Autodesk Inventor part; units mm, degrees
ref_plane "Work Plane1" through (0, 20, 0) normal (0, -1, 0) x (1, 0, 0)
ref_plane "YZ Plane" through (0, 0, 0) normal (1, 0, 0) x (0, 1, 0)
ref_plane "XZ Plane" through (0, 0, 0) normal (0, 1, 0) x (-1, 0, 0)
sketch "Sketch1" plane through (0, 0, 0) normal (0, 1, 0) x (-1, 0, 0)
  line L0 (-19.05, -19.05) -> (19.05, -19.05) construction
  line L1 (19.05, -19.05) -> (19.05, 19.05) construction
  line L2 (19.05, 19.05) -> (-19.05, 19.05) construction
  line L3 (-19.05, 19.05) -> (-19.05, -19.05) construction
  line L4 (-19.05, -19.05) -> (19.05, 19.05) construction
  line L5 (19.05, -19.05) -> (-19.05, 19.05) construction
  line L6 (-19.05, 19.05) -> (19.05, 19.05) construction
  line L7 (19.05, 19.05) -> (19.05, 39.05) construction
  line L8 (19.05, 39.05) -> (-19.05, 39.05)
  line L9 (-19.05, 39.05) -> (-19.05, 19.05) construction
  line L10 (19.05, 39.05) -> (39.05, 39.05)
  line L11 (39.05, 39.05) -> (39.05, -19.05)
  line L12 (39.05, -19.05) -> (19.05, -19.05) construction
  line L13 (19.05, -19.05) -> (19.05, 19.05) construction
  line L14 (19.05, 19.05) -> (19.05, 39.05) construction
  line L15 (-19.05, 39.05) -> (39.05, 39.05)
  line L16 (45.4, 39.05) -> (45.4, 45.4)
  line L17 (45.4, 45.4) -> (-19.05, 45.4)
  line L18 (-19.05, 45.4) -> (-19.05, 39.05)
  line L19 (45.4, 39.05) -> (39.05, 39.05) construction
  line L20 (39.05, 39.05) -> (39.05, -19.05)
  line L21 (39.05, -19.05) -> (45.4, -19.05)
  line L22 (45.4, -19.05) -> (45.4, 39.05)
  line L23 (39.05, 39.05) -> (45.4, 39.05) construction
  point P0 (0, 0)
  dimension "d0" = 38.1
  dimension "d1" = 20
  dimension "d2" = 20
  dimension "d3" = 6.35
  dimension "d4" = 6.35
  dimension "d67" = 0
extrude "Extrusion1" add sketch "Sketch1" along normal blind 62.3
sketch "Sketch2" plane through (-45.4, 0, 45.4) normal (0, 0, 1) x (1, 0, 0)
  line L0 (6.35, 0) -> (0, 0)
  line L1 (64.45, 0) -> (64.45, 62.3)
  line L2 (0, 0) -> (64.45, 0)
  line L3 (64.45, 0) -> (64.45, 20)
  line L4 (64.45, 20) -> (0, 20)
  line L5 (0, 20) -> (0, 0)
  line L6 (0, 0) -> (0, 62.3)
  line L7 (0, 10) -> (64.45, 10) construction
  circle A0 centre (19.05, 10) radius 2.75
  circle A1 centre (35.4, 10) radius 2.75
  circle A2 centre (51.75, 10) radius 2.75
  point P0 (45.4, 0)
  dimension "d7" = 20
  dimension "d8" = 5.5
  dimension "d12" = 16.35
  dimension "d68" = 12.7
extrude "Extrusion2" cut sketch "Sketch2" against normal blind 62.3 contours A0 | A1 | A2
sketch "Sketch3" plane through (-45.4, 0, -19.05) normal (-1, 0, 0) x (0, 0, 1)
  circle A0 centre (12.7, 10) radius 2.75
  line L0 (0, 0) -> (64.45, 0)
  line L1 (0, 0) -> (0, 62.3)
  circle A1 centre (29.05, 10) radius 2.75
  circle A2 centre (45.4, 10) radius 2.75
  point P0 (19.05, 0)
  dimension "d19" = 10
  dimension "d20" = 5.5
  dimension "d21" = 12.7
  dimension "d24" = 16.35
extrude "Extrusion3" cut sketch "Sketch3" against normal blind 62.3
ref_plane "Work Plane1" through (0, 20, 0) normal (0, -1, 0) x (1, 0, 0)
sketch "Sketch4" plane through (0, 20, 0) normal (0, -1, 0) x (1, 0, 0)
  line L0 (-39.05, -19.05) -> (-45.4, -19.05)
  line L1 (-39.05, 39.05) -> (-39.05, -19.05)
  line L2 (19.05, 39.05) -> (-39.05, 39.05)
  line L3 (19.05, 45.4) -> (19.05, 39.05)
  line L4 (-45.4, 45.4) -> (19.05, 45.4)
  line L5 (-45.4, -19.05) -> (-45.4, 45.4)
  line L6 (-39.05, 39.05) -> (-39.05, -19.05)
  line L7 (-39.05, 39.05) -> (-19.05, 39.05)
  line L8 (-19.05, 39.05) -> (-19.05, 19.05) construction
  line L9 (-19.05, -19.05) -> (-39.05, -19.05)
  line L10 (-39.05, -19.05) -> (-39.05, 39.05)
  line L11 (19.05, 39.05) -> (-39.05, 39.05)
  line L12 (19.05, 39.05) -> (-19.05, 39.05)
  line L13 (-19.05, 39.05) -> (-19.05, 19.05) construction
  line L14 (-19.05, 19.05) -> (19.05, 19.05) construction
  line L15 (19.05, 19.05) -> (19.05, 39.05)
  line L16 (-19.05, 19.05) -> (-19.05, -19.05) construction
  line L17 (19.05, 29.05) -> (-39.05, 29.05) construction
  line L18 (-29.05, -19.05) -> (-29.05, 39.05) construction
  circle A0 centre (-29.05, 29.05) radius 2.75
  circle A1 centre (-10, 29.05) radius 2.75
  circle A2 centre (9.05, 29.05) radius 2.75
  circle A3 centre (-29.05, 10) radius 2.75
  circle A4 centre (-29.05, -9.05) radius 2.75
  line L19 (19.05, 19.05) -> (19.05, 12.7)
  line L20 (19.05, 12.7) -> (-19.05, -19.05)
  circle A5 centre (-29.05, 4.126) radius 2.7544
  point P0 (0, 0)
  dimension "d32" = 20
  dimension "d35" = 19.05
  dimension "d40" = 5.5
  dimension "d43" = 19.05
  dimension "d50" = 6.35
  dimension "d69" = 0
extrude "Extrusion4" add sketch "Sketch4" against normal blind 6.35 contours L1 L2 L15 L19 L20 L9 | A3
sketch "Sketch5" plane through (0, 26.35, 0) normal (0, 1, 0) x (1, 0, 0)
  line L0 (19.05, -39.05) -> (19.05, -12.7)
  line L1 (-39.05, -39.05) -> (-39.05, 19.05)
  line L2 (19.05, -12.7) -> (-39.05, -12.7)
  line L3 (-39.05, -12.7) -> (-39.05, -19.05)
  line L4 (-39.05, -19.05) -> (19.05, -19.05)
  line L5 (19.05, -19.05) -> (19.05, -12.7)
  point P0 (0, 0)
  dimension "d51" = 6.35
extrude "Extrusion5" add sketch "Sketch5" along normal up to surface (35.95 mm away)
sketch "Sketch7" plane through (-39.05, 26.35, -19.05) normal (1, 0, 0) x (0, 0, -1)
  line L0 (-31.75, 35.95) -> (0, 35.95)
  line L1 (-31.75, 35.95) -> (0, 35.95)
  line L2 (0, 0) -> (0, 35.95)
  line L3 (0, 35.95) -> (0, 0)
  line L4 (0, 0) -> (-31.75, 35.95)
  point P0 (-19.05, -26.35)
extrude "Extrusion7" cut sketch "Sketch7" against normal through all
sketch "Sketch8" plane through (-45.4, 0, 45.4) normal (0, 0, 1) x (1, 0, 0)
  line L0 (64.45, 62.3) -> (6.35, 62.3)
  line L1 (6.35, 26.35) -> (6.35, 62.3)
  line L2 (64.45, 26.35) -> (6.35, 26.35)
  line L3 (64.45, 26.35) -> (64.45, 62.3)
  line L4 (64.45, 20) -> (64.45, 26.35)
  line L5 (6.35, 62.3) -> (64.45, 26.35)
  line L6 (6.35, 62.3) -> (64.45, 62.3)
  line L7 (64.45, 26.35) -> (64.45, 62.3)
  line L8 (64.45, 62.3) -> (6.35, 62.3)
  point P0 (45.4, 0)
extrude "Extrusion8" cut sketch "Sketch8" against normal through all contours L3 L5 L0
sketch "Sketch9" plane through (-39.05, 26.35, 39.05) normal (1, 0, 0) x (0, 0, -1)
  line L0 (12.75, -6.35) -> (7.25, -6.35)
  line L1 (10, -6.35) -> (10, 18.61)
  circle A0 centre (10, 18.61) radius 2.75
  point P0 (39.05, -26.35)
  dimension "d63" = 24.96
  dimension "d64" = 5.5
extrude "Extrusion9" cut sketch "Sketch9" against normal through all
properties part number "xIdler"
The model under review builds one solid part; all positions refer to its coordinate system, in mm. A direction names the side the tool comes from. Give positions to 0.01 mm unless a question says otherwise; leave off trailing zeros. Write each loop counter-clockwise with the first axis right and the second up, starting at its lowest first coordinate (ties: lowest second). Pieces come first, ordered by that corner, then holes. Notation, with made-up numbers: M 48,24 L 89,24 A26 cw 89,43 Z; hole C -18.5,89 d8. An arc over 180 degrees is marked long. Write each question's results on one line, items separated by ' | '. Start each with the question number.
1. We need section D-D (x = -22.5). Write out the cut boundary in (y, z).
2. We need section B-B (y = 24). Write out the cut boundary in (x, z), and give its area (3 significant figures).
3. We need section C-C (y = 15.5). Write out the cut boundary in (x, z), and give its area (3 significant figures).
4. We need section A-A (z = -10). Write out the cut boundary in (x, y), and give its area (3 significant figures).
5. Mouldability with a two-part tool opening along Z and no side actions: class faces 5 (the flat face through (-25, 0, 40)), 6 (the flat face through (-23, 36, 12.7)), 7 (the cylindrical face through (-8.52, 23.13, 31.37)) as released by +Z, released by -Z, zero draft, split by the parting line, or undercut.
6. For probe 1 along Z at (x, y) = (-29.05, 23.75); probe 2 along X at (y, z) = (22, 29); probe 3 along Z at (x, y) = (-19.5, 31), list the stretches that pass through material, from the lowest coordinate up. Write a range as [from, to].
7. Insertion check: pin 1 Ø3.5 at (x, z) = (-10, 29.05) entering from +Y; pin 2 Ø10 at (x, z) = (-18, 4) entering from -Y; pin 3 Ø16 at (y, z) = (13, -1) entering from +X; pin 4 Ø6.5 at (x, z) = (-29.05, 29.05) entering from +Y. Each pin has a flat end and moves straight along its axis. Give the tip position at first contact, or say it passes through.
8. For faces 1 (the flat face through (-39.05, 40, 29)), 2 (the flat face through (-39.05, 40, 1)), 3 (the flat face through (-10, 5, 39.05)), 4 (the flat face through (-10.41, 44.58, 15.92)), list the 3-axis set-ups (+Z, -Z, +X, -X, +Y, -Y) from which the entire face can be reached by the end or side of a thin tool; tool diameter is ignored.
Results found:
1) outline: M 0,39.05 L 20,39.05 L 20,-19.05 L 26.35,-19.05 L 26.35,12.7 L 52.06,12.7 L 52.06,19.05 L 26.35,19.05 L 26.35,39.05 L 52.06,39.05 L 52.06,45.4 L 0,45.4 Z
2) outline: M -45.4,-19.05 L -19.05,-19.05 L 19.05,12.7 L 19.05,45.4 L -45.4,45.4 Z; hole C -29.05,-9.05 d5.5; hole C -29.05,4.13 d5.51; hole C -29.05,29.05 d5.5; hole C -10,29.05 d5.5; hole C 9.05,29.05 d5.5 | area: 3,430 mm^2
3) outline: M -45.4,-19.05 L -39.05,-19.05 L -39.05,39.05 L 19.05,39.05 L 19.05,45.4 L -45.4,45.4 Z | area: 778 mm^2
4) outline: M -45.4,0 L -39.05,0 L -39.05,20 L -31.63,20 L -31.63,26.35 L -39.05,26.35 L -39.05,36.6 L -45.4,36.6 Z; M -26.47,20 L -8.19,20 L -8.19,26.35 L -26.47,26.35 Z | area: 396 mm^2
5) face 5: zero draft | face 6: released by -Z | face 7: undercut
6) probe 1: z = [-19.05, -11.8], [-6.3, 1.37], [6.88, 26.3], [31.8, 45.4] | probe 2: x = [-45.4, -31.8], [-26.3, -12.75], [-7.25, 6.3], [11.8, 19.05] | probe 3: z = [12.7, 19.05], [39.05, 45.4]
7) pin 1: passes through | pin 2: stops at y = 20 | pin 3: stops at x = 7.26 | pin 4: stops at y = 26.35
8) face 1: +X, +Y | face 2: -Z, +X, +Y | face 3: -Z, +X, -Y | face 4: +Z, -Z, +X, +Y
